from build123d import *

# Parameters (mm, degrees)
F0_W     = 55
F0_H     = 100
F1_DEPTH = 3
F2_R     = 21
F3_DEPTH = 272
F4_R     = 6.35
F5_DEPTH = 30
F4_R_2   = 9.525
F6_DEPTH = 40


# Not quite as in the source:
# - a feature names something its author has since deleted; it is built from what else it names


with BuildPart() as f1:
    # F0 (on Front) → F1 (new body)
    with BuildSketch(Plane.XZ):
        Rectangle(F0_W, F0_H)
        with BuildLine():
            ThreePointArc((-10, -35), (-8.5355339059, -31.4644660941), (-5, -30))
            Line((-5, -30), (0, -30))
            Line((0, -30), (5, -30))
            ThreePointArc((5, -30), (8.5355339059, -31.4644660941), (10, -35))
            ThreePointArc((10, -35), (8.5355339059, -38.5355339059), (5, -40))
            Line((5, -40), (0, -40))
            Line((0, -40), (-5, -40))
            ThreePointArc((-5, -40), (-8.5355339059, -38.5355339059), (-10, -35))
        make_face(mode=Mode.SUBTRACT)
        with BuildLine():
            Line((-5, 30), (-5, 40))
            ThreePointArc((-5, 40), (0, 45), (5, 40))
            Line((5, 40), (5, 30))
            ThreePointArc((5, 30), (0, 25), (-5, 30))
        make_face(mode=Mode.SUBTRACT)
    extrude(amount=F1_DEPTH)

    # F2 (on face) → F3 (join)
    with BuildSketch(Plane.XZ.offset(3)):
        Circle(F2_R)
    extrude(amount=F3_DEPTH)

    # F4 (on Top) → F5 (join)
    with BuildSketch(Plane.XY):
        with Locations((0, -41)):
            Circle(F4_R)
    extrude(amount=-F5_DEPTH)

    # F4 (on Top) → F6 (join)
    with BuildSketch(Plane.XY):
        with Locations((0, -236)):
            Circle(F4_R_2)
    extrude(amount=-F6_DEPTH)


solid = f1.part
Can you work these out from the model? Positions are in its coordinate system, mm. A direction names the side the tool comes from. Coordinates: 2 decimals unless noted, no trailing zeros. Write each loop counter-clockwise with the first axis right and the second up, starting at its lowest first coordinate (ties: lowest second). Pieces come first, ordered by that corner, then holes. Notation, with made-up numbers: (-32, 40.25) -> (21, 40.25) arc R24 ccw to (21, 56.25) -> close; hole circle Ø8 at (-18, 39.25). An arc over 180 degrees is marked (long way). Write item = value, one per line.
(1) On a 3-axis mill with a long thin cutter (end or side, diameter ignored), from which of +Z, -Z, +X, -X, +Y, -Y can I reach the whole of each face in a straight line? I mean faces 1 (the face through (0, -1, 25)), 2 (the face through (-2.06, -245.3, -29.21)). Say none if no direction works.
Verdict:
face_1 = +Y, -Y
face_2 = -Z
(2) Imagine slicing it at D-D (y = -236). Please give me the cut outline in (x, z) (3 decimals).
Verdict:
outline = (-9.525, -40) -> (9.525, -40) -> (9.525, -18.716) arc R21 ccw (long way) to (-9.525, -18.716) -> close
(3) Thinking about a two-plate mould opening in Z: for faces 3 (the face through (-6.344, -40.721, -24.939)), 4 (the face through (0, -1, 45)), 5 (the face through (0, -236, -40)), which applies, +Z half, -Z half, draft (parallel to the pull), parting line (faces both ways), or undercut?
Verdict:
face_3 = draft
face_4 = undercut
face_5 = -Z half
(4) For pin 1 (12 mm diameter, centred on y = -194.5, z = 20, fed in from -X); pin 2 (4 mm diameter, centred on x = -2.5, y = -40, fed in from -Z); pin 3 (8 mm diameter, centred on x = -10, y = -159, fed in from +Z), each with a flat end and sliding along its axis, tell me the tip position at first contact or that it passes through.
Verdict:
pin_1 = -15.65
pin_2 = -30
pin_3 = 20.12
(5) Imagine slicing it at C-C (x = -16). Please give me the cut outline in (y, z), and give its area (3 significant figures).
Verdict:
outline = (-275, -13.6) -> (-3, -13.6) -> (-3, -50) -> (0, -50) -> (0, 50) -> (-3, 50) -> (-3, 13.6) -> (-275, 13.6) -> close
area = 7,700 mm^2
(6) If I drill on probe 1 along Y at (x, z) = (-24, 1); probe 2 along Z at (x, y) = (1, -179); probe 3 along Z at (x, y) = (-16.5, -246.5), over which ranges is the centre line in solid material (lowest first)?
Verdict:
probe_1 = -3 to 0
probe_2 = -20.98 to 20.98
probe_3 = -12.99 to 12.99
(7) Imagine slicing it at B-B (y = -28.5). Please give me the cut outline in (x, z).
Verdict:
outline = circle Ø42 at (0, 0)
(8) Imagine slicing it at A-A (z = 0). Please give me the cut outline in (x, y).
Verdict:
outline = (-27.5, -3) -> (-21, -3) -> (-21, -275) -> (21, -275) -> (21, -3) -> (27.5, -3) -> (27.5, 0) -> (-27.5, 0) -> close
